from build123d import *

# Parameters (mm, degrees)
BOSS_EXTRUDE2_DEPTH     = 12
SKETCH5_R               = 1.65
CUT_EXTRUDE3_DEPTH      = 6
SKETCH6_W               = 12
SKETCH6_H               = 6.5
CUT_EXTRUDE4_DEPTH      = 13
SKETCH8_W               = 64
SKETCH8_H               = 8
BOSS_EXTRUDE3_DEPTH     = 5
SKETCH11_R              = 1.65
CUT_EXTRUDE7_DEPTH      = 76.896039473
SKETCH13_R              = 21.1
CUT_EXTRUDE8_DEPTH      = 21
CUT_EXTRUDE9_DEPTH      = 71.896039473
CUT_EXTRUDE9_DEPTH_BACK = 10


with BuildPart() as part:
    # Sketch1 → Boss-Extrude2 (new body)
    with BuildSketch(Plane.XY):
        with BuildLine():
            Line((0, 0), (64, 0))
            Line((64, 0), (71.941945847, 6.076635266))
            Line((71.941945847, 6.076635266), (89.619615377, 23.754304796))
            ThreePointArc((89.619615377, 23.754304796), (95.283552654, 63.552389681), (55.861435714, 71.4177849))
            Line((55.861435714, 71.4177849), (-7.778174593, 7.778174593))
            Line((-7.778174593, 7.778174593), (0, 0))
        make_face()
    extrude(amount=BOSS_EXTRUDE2_DEPTH)

    # Sketch5 → Cut-Extrude3 (cut)
    with BuildSketch(Plane.XZ):
        with Locations((11.5, 6)):
            Circle(SKETCH5_R)
        with Locations((52.5, 6)):
            Circle(SKETCH5_R)
    extrude(amount=-CUT_EXTRUDE3_DEPTH, mode=Mode.SUBTRACT)

    # Sketch6 → Cut-Extrude4 (cut, through all)
    with BuildSketch(Plane.XY.offset(12)):
        with Locations((12, 9.25)):
            Rectangle(SKETCH6_W, SKETCH6_H)
        with Locations((52, 9.25)):
            Rectangle(SKETCH6_W, SKETCH6_H)
    extrude(amount=-CUT_EXTRUDE4_DEPTH, mode=Mode.SUBTRACT)

    # Sketch8 → Boss-Extrude3 (add)
    with BuildSketch(Plane.XZ):
        with Locations((32, -4)):
            Rectangle(SKETCH8_W, SKETCH8_H)
    extrude(amount=-BOSS_EXTRUDE3_DEPTH)

    # Sketch11 → Cut-Extrude7 (cut, through all)
    with BuildSketch(Plane.XZ):
        with Locations((11.5, -4)):
            Circle(SKETCH11_R)
        with Locations((52.5, -4)):
            Circle(SKETCH11_R)
    extrude(amount=-CUT_EXTRUDE7_DEPTH, mode=Mode.SUBTRACT)

    # Sketch13 → Cut-Extrude8 (cut, through all)
    with BuildSketch(Plane.XY.offset(12)):
        with Locations((71.414976798, 46.64721049)):
            Circle(SKETCH13_R)
    extrude(amount=-CUT_EXTRUDE8_DEPTH, mode=Mode.SUBTRACT)

    # Sketch15 → Cut-Extrude9 (cut, two sides)
    with BuildSketch(Plane(origin=(0, 5, 0), x_dir=(1, 0, 0), z_dir=(0, 1, 0))) as cut_extrude9_sk:
        with BuildLine():
            Line((45, 8), (19, 8))
            ThreePointArc((19, 8), (32, 2.615223689), (45, 8))
        make_face()
    extrude(amount=CUT_EXTRUDE9_DEPTH, mode=Mode.SUBTRACT)
    extrude(cut_extrude9_sk.sketch, amount=-CUT_EXTRUDE9_DEPTH_BACK, mode=Mode.SUBTRACT)


solid = part.part
Read the model definition and answer for the solid it produces. Units are mm, in the model's axes. A direction names the side the tool comes from. Round coordinates to 2 decimals unless told otherwise and drop trailing zeros. Loops run counter-clockwise (first coordinate to the right, second up) from the corner with the lowest first, then second, coordinate; pieces in that order, holes last.
Q1. Each of these flat-tipped pins is pushed along its axis until it touches: pin 1 (2.5 mm diameter, centred on y = 3, z = -3.5, fed in from +X); pin 2 (1.5 mm diameter, centred on x = 85.5, z = 9, fed in from -Y); pin 3 (6 mm diameter, centred on x = 13.5, z = 4, fed in from +Y). Where does it stop, or does it pass through?
Q2. Determine the mould class of faces 1 (the face through (46, 30, 12)), 2 (the face through (91.54, 52.99, 6.08)), 3 (the face through (13.024, 2.465, -4.632)), 4 (the face through (13.024, 2.958, 5.368)) for opening direction Z: released by +Z, released by -Z, zero draft, split by the parting line, or undercut.
Q3. Section B-B on y = 66 is taken. Write down the section's boundary in (x, z), and give its area (3 significant figures).
Q4. Section C-C on x = 61 is taken. Write down the section's boundary in (y, z), and give its area (3 significant figures).
Q5. Section A-A on z = -4 is taken. Write down the section's boundary in (x, y), and give its area (3 significant figures).
Q6. Consider probe 1 along Z at (x, y) = (52.5, 3); probe 2 along Z at (x, y) = (23.5, 10.5); probe 3 along Y at (x, z) = (87.5, 10). Determine where each line is inside the solid, lowest interval first.
Q7. Which of the six approach directions +Z, -Z, +X, -X, +Y, -Y give full straight-line access (tool end or side, diameter ignored) to faces 5 (the face through (0, 2, -4)), 6 (the face through (80.657, 14.792, 5.916)), 7 (the face through (64, 2, -4)), 8 (the face through (6, 9, 6))?
Q8. Section D-D on x = 11.5 is taken. Write down the section's boundary in (y, z), and give its area (3 significant figures).
Output:
1. pin 1: stops at x = 64
1. pin 2: stops at y = 18.88
1. pin 3: stops at y = 32.06
2. face 1: released by +Z
2. face 2: zero draft
2. face 3: undercut
2. face 4: undercut
3. outline: (50.44, 0) - (63.01, 0) - (63.01, 12) - (50.44, 12) - close; (79.82, 0) - (93.35, 0) - (93.35, 12) - (79.82, 12) - close
3. area: 313 mm2
4. outline: (0, -8) - (5, -8) - (5, 0) - (28.3, 0) - (28.3, 12) - (0, 12) - close; (65, 0) - (73.98, 0) - (73.98, 12) - (65, 12) - close
4. area: 487 mm2
5. outline: (0, 0) - (9.85, 0) - (9.85, 5) - (0, 5) - close; (13.15, 0) - (25, 0) - (25, 5) - (13.15, 5) - close; (39, 0) - (50.85, 0) - (50.85, 5) - (39, 5) - close; (54.15, 0) - (64, 0) - (64, 5) - (54.15, 5) - close
5. area: 217 mm2
6. probe 1: z = -8 to -5.65, -2.35 to 4.35, 7.65 to 12
6. probe 2: z = 0 to 12
6. probe 3: y = 21.63 to 32.99, 60.3 to 71.08
7. face 5: -Z, -X, +Y, -Y
7. face 6: +Z, -Z, +X, -Y
7. face 7: -Z, +X, +Y, -Y
7. face 8: +Z, -Z
8. outline: (0, -8) - (5, -8) - (5, -5.65) - (0, -5.65) - close; (0, -2.35) - (5, -2.35) - (5, 0) - (6, 0) - (6, 4.35) - (0, 4.35) - close; (0, 7.65) - (6, 7.65) - (6, 12) - (0, 12) - close; (12.5, 0) - (27.06, 0) - (27.06, 12) - (12.5, 12) - close
8. area: 250 mm2
